from build123d import *

# Parameters (mm, degrees)
F0_R     = 3.75
F1_DEPTH = 2.6
F2_R     = 2
F3_DEPTH = 15
F4_SIZE  = 0.5
F6_DEPTH = 1.95
F7_R     = 2.3


with BuildPart() as f1:
    # F0 (on Right) → F1 (new body)
    with BuildSketch(Plane.YZ):
        Circle(F0_R)
    extrude(amount=-F1_DEPTH)

    # F2 (on face) → F3 (join)
    with BuildSketch(Plane(origin=(-2.6, 0, 0), x_dir=(0, -1, 0), z_dir=(-1, 0, 0))):
        Circle(F2_R)
    extrude(amount=F3_DEPTH)

    # F4
    f4_edges = [f1.edges().sort_by_distance(p)[0] for p in [
        (-17.6, 2, 0),
    ]]
    chamfer(f4_edges, length=F4_SIZE)

    # F5 (on face) → F6 (cut)
    with BuildSketch(Plane.YZ):
        Polygon((0, -1.443376), (1.25, -0.721688), (1.25, 0.721688), (0, 1.443376), (-1.25, 0.721688), (-1.25, -0.721688), align=None)
    extrude(amount=-F6_DEPTH, mode=Mode.SUBTRACT)

    # F7
    f7_edges = [f1.edges().sort_by_distance(p)[0] for p in [
        (0, -3.75, 0),
    ]]
    fillet(f7_edges, radius=F7_R)


solid = f1.part
Check sheet for the modelled part. Datum: model origin and axes. Units: mm. A direction names the side the tool comes from. Round coordinates to 2 decimals unless told otherwise and drop trailing zeros. Order: outer loops, then holes, each group sorted by start corner. A loop starts at its lowest first (then second) coordinate and runs counter-clockwise, first axis right, second up.
(1) Go/stop test with flat-tipped pins: P1, Ø3, axis at x = -11, y = -0.5, coming from the +Z side; P2, Ø0.7, axis at x = -1, z = 0, coming from the -Y side; P3, Ø4, axis at x = -12.5, y = 1, coming from the -Z side. Record where each tip stops, or that it passes through.
(2) Scan lines: probe 1 along X at (y, z) = (-0.5, 0.25); probe 2 along Z at (x, y) = (-10.75, 0); probe 3 along X at (y, z) = (-0.75, 3). Record each from-to range of solid material in increasing order.
(3) Draft check along Z on faces 3 (the flat face through (-17.6, 0, 0)), 4 (the flat face through (-0.96, -0.63, -1.08)), 5 (the cylindrical face through (-10, 0, -2)). Enter one of: pulls with the +Z half, pulls with the -Z half, needs draft (parallel to the pull), parting line crosses it, or undercut.
(4) Cross-section at A-A, the plane x = -7.5. Enter the section's corners in (y, z), and give its area (3 significant figures).
(5) Access from +Z, -Z, +X, -X, +Y, -Y to the whole of each face (thin tool, end or side, straight path). Record for faces 1 (the flat face through (-2.6, 2, -2)), 2 (the flat face through (-0.961, 0.616, -1.088)).
Check sheet entries:
1. P1: stops at z = 2
1. P2: stops at y = -3.54
1. P3: stops at z = -2
2. probe 1: x = -17.6 to -1.95
2. probe 2: z = -2 to 2
2. probe 3: x = -2.6 to -0.69
3. face 3: needs draft
3. face 4: undercut
3. face 5: parting line crosses it
4. outline: circle Ø4 at (0, 0)
4. area: 12.6 mm2
5. face 1: -X
5. face 2: +X
